from build123d import *

# Parameters (mm, degrees)
SKETCH_W     = 70
SKETCH_H     = 70
PAD_DEPTH    = 12
SKETCH001_W  = 45.72
SKETCH001_H  = 40.64
POCKET_DEPTH = 6
FILLET_R     = 0.2
FILLET001_R  = 1
SKETCH002_R  = 1.5
HOLE_DEPTH   = 25


with BuildPart() as part:
    # Sketch → Pad (new body)
    with BuildSketch(Plane.XY):
        Rectangle(SKETCH_W, SKETCH_H)
    extrude(amount=PAD_DEPTH)

    # Sketch001 (on Face6 of Pad) → Pocket (cut)
    with BuildSketch(Plane.XY.offset(12)):
        with Locations((0, -0.01)):
            Rectangle(SKETCH001_W, SKETCH001_H)
    extrude(amount=-POCKET_DEPTH, mode=Mode.SUBTRACT)

    # Fillet
    fillet_edges = [part.edges().sort_by_distance(p)[0] for p in [
        (-22.86, -20.33, 9),
    ]]
    fillet(fillet_edges, radius=FILLET_R)

    # Fillet001
    fillet001_edges = [part.edges().sort_by_distance(p)[0] for p in [
        (-22.86, 0.09, 12),
        (-22.801421, -20.271421, 12),
        (0, 20.31, 12),
        (0.1, -20.33, 12),
        (22.86, -0.01, 12),
        (0, 35, 12),
        (-35, 0, 12),
        (35, 0, 12),
        (0, -35, 12),
        (-22.86, -20.13, 9),
        (-22.86, 20.31, 9),
        (-22.86, 0.09, 6),
        (-22.66, -20.33, 9),
        (-22.801421, -20.271421, 6),
        (22.86, 20.31, 9),
        (0, 20.31, 6),
        (22.86, -20.33, 9),
        (0.1, -20.33, 6),
        (22.86, -0.01, 6),
        (-35, 35, 6),
        (35, 35, 6),
        (0, 35, 0),
        (-35, -35, 6),
        (-35, 0, 0),
        (35, -35, 6),
        (35, 0, 0),
        (0, -35, 0),
    ]]
    fillet(fillet001_edges, radius=FILLET001_R)

    # Sketch002 (on Face11 of Fillet) → Hole (cut)
    with BuildSketch(Plane.XY.offset(6)):
        with Locations((-20.32, 17.78)):
            Circle(SKETCH002_R)
        with Locations((20.32, -17.78)):
            Circle(SKETCH002_R)
    extrude(amount=-HOLE_DEPTH, mode=Mode.SUBTRACT)


solid = part.part
Source: CAD feature listing. Evaluate the final solid. Frame: model axes, mm. A direction names the side the tool comes from. Give positions to 0.01 mm unless a question says otherwise; leave off trailing zeros. Order: outer loops, then holes, each group sorted by start corner. A loop starts at its lowest first (then second) coordinate and runs counter-clockwise, first axis right, second up. Notation, with made-up numbers: (35.25, 80.5) -> (78.25, 80.5) arc R21 ccw to (78.25, 109.5) -> close; hole circle Ø4 at (-30.75, 58.25). An arc over 180 degrees is marked (long way). Write item = value, one per line.
Item 1: Section query C-C (x = 11.5). Output: boundary loops of the cut face in (y, z), then the cut area to 3 significant figures.
Check result:
outline = (-35, 1) arc R1 ccw to (-34, 0) -> (34, 0) arc R1 ccw to (35, 1) -> (35, 11) arc R1 ccw to (34, 12) -> (21.31, 12) arc R1 ccw to (20.31, 11) -> (20.31, 7) arc R1 cw to (19.31, 6) -> (-19.33, 6) arc R1 cw to (-20.33, 7) -> (-20.33, 11) arc R1 ccw to (-21.33, 12) -> (-34, 12) arc R1 ccw to (-35, 11) -> close
area = 595 mm²
Item 2: Section query D-D (y = 4). Output: boundary loops of the cut face in (x, z).
Check result:
outline = (-35, 1) arc R1 ccw to (-34, 0) -> (34, 0) arc R1 ccw to (35, 1) -> (35, 11) arc R1 ccw to (34, 12) -> (23.86, 12) arc R1 ccw to (22.86, 11) -> (22.86, 7) arc R1 cw to (21.86, 6) -> (-21.86, 6) arc R1 cw to (-22.86, 7) -> (-22.86, 11) arc R1 ccw to (-23.86, 12) -> (-34, 12) arc R1 ccw to (-35, 11) -> close
Item 3: Set-up query: faces 1 (the face through (0, 0, 0)), 2 (the face through (0, 0, 6)). Return all of +Z, -Z, +X, -X, +Y, -Y with unobstructed straight access to the full face (end or side cutting, diameter ignored); none if empty.
Check result:
face_1 = -Z, +X, -X, +Y, -Y
face_2 = +Z
Item 4: Mould query, pull axis Y, two halves, no side actions, for faces 3 (the face through (0, 23, 12)), 4 (the face through (-22.86, -1, 9)), 5 (the face through (0, -35, 6)), 6 (the face through (-19.63, 16.45, 3.04)). Classes: +Y half, -Y half, draft (parallel to the pull), parting line (faces both ways), or undercut.
Check result:
face_3 = draft
face_4 = undercut
face_5 = -Y half
face_6 = undercut
Item 5: Ray query, probe 1 along Y at (x, z) = (-20.32, 2.35); probe 2 along Y at (x, z) = (20.32, 3.05); probe 3 along Z at (x, y) = (-17, 7.5). Return the intervals inside material, ascending.
Check result:
probe_1 = -35 to 16.28, 19.28 to 35
probe_2 = -35 to -19.28, -16.28 to 35
probe_3 = 0 to 6
Item 6: Contact query for flat-ended pins moving along their axis: pin 1 (8 mm diameter, centred on x = -21.5, y = 0.5, fed in from +Z); pin 2 (2.5 mm diameter, centred on x = -20.32, y = 17.78, fed in from +Z); pin 3 (1.5 mm diameter, centred on x = -9, y = -1.5, fed in from +Z). Output: stop coordinate, or through.
Check result:
pin_1 = 12
pin_2 = through
pin_3 = 6
Item 7: Section query B-B (x = 20.32). Output: boundary loops of the cut face in (y, z).
Check result:
outline = (-35, 1) arc R1 ccw to (-34, 0) -> (-19.28, 0) -> (-19.28, 6) -> (-19.33, 6) arc R1 cw to (-20.33, 7) -> (-20.33, 11) arc R1 ccw to (-21.33, 12) -> (-34, 12) arc R1 ccw to (-35, 11) -> close; (-16.28, 0) -> (34, 0) arc R1 ccw to (35, 1) -> (35, 11) arc R1 ccw to (34, 12) -> (21.31, 12) arc R1 ccw to (20.31, 11) -> (20.31, 7) arc R1 cw to (19.31, 6) -> (-16.28, 6) -> close
